Read the model definition and answer for the solid it produces. Units are mm, in the model's axes. A direction names the side the tool comes from. Coordinates: 2 decimals unless noted, no trailing zeros. Loops run counter-clockwise (first coordinate to the right, second up) from the corner with the lowest first, then second, coordinate; pieces in that order, holes last. Notation, with made-up numbers: (-33.5, 58.25) -> (-0.5, 58.25) arc R19 cw to (-0.5, 91.25) -> close; hole circle Ø3 at (71.25, -14). An arc over 180 degrees is marked (long way). Answer as a JSON object with one key per item and string values. Group by question number.
1) Section C-C, the plane z = -61 is taken. Give the vertices of the cut face in (x, y).
2) Section A-A, the plane y = 6 is taken. Give the vertices of the cut face in (x, z).
3) Which of the six approach directions +Z, -Z, +X, -X, +Y, -Y give full straight-line access (tool end or side, diameter ignored) to faces 1 (the face through (17.656, 4.824, -16.21)), 2 (the face through (20.344, 4.824, -17.79)), 3 (the face through (20.344, 4.824, -50.79))?
4) Determine the mould class of faces 4 (the face through (28, 0, -33)), 5 (the face through (17.644, 4.824, -17.768)), 6 (the face through (17.644, 4.824, -50.768)) for opening direction Z: released by +Z, released by -Z, zero draft, split by the parting line, or undercut.
5) Section B-B, the plane x = 19 is taken. Give the vertices of the cut face in (y, z), plus the area to 3 significant figures.
6) Flat-ended cylindrical pins translate along their axes: P1, Ø0.5, axis at x = 18.5, y = 5, coming from the -Z side; P2, Ø0.9, axis at x = 19, y = 4, coming from the +Z side. Find the tip coordinate at first contact, or state that the pin passes through.
7) Consider probe 1 along Y at (x, z) = (51, -59); probe 2 along X at (y, z) = (3.5, -18.5). Determine where each line is inside the solid, lowest interval first. Write a range as [from, to].
8) Section D-D, the plane x = 13.5 is taken. Give the vertices of the cut face in (y, z), plus the area to 3 significant figures.
Autodesk Inventor part; units mm, degrees
ref_plane "YZ Plane" through (0, 0, 0) normal (1, 0, 0) x (0, 1, 0)
ref_plane "XZ Plane" through (0, 0, 0) normal (0, 1, 0) x (-1, 0, 0)
ref_plane "XY Plane" through (0, 0, 0) normal (0, 0, 1) x (1, 0, 0)
sketch "Sketch1" plane through (0, 0, 0) normal (0, 1, 0) x (-1, 0, 0)
  line L0 (0, 0) -> (-55, 0)
  line L1 (-55, 0) -> (-55, -67)
  line L2 (-55, -67) -> (0, -67)
  line L3 (0, -67) -> (0, 0)
  dimension "d0" = 55
  dimension "d1" = 67
extrude "Extrusion1" add sketch "Sketch1" along normal blind 3
sketch "Sketch2" plane through (0, 3, 0) normal (0, 1, 0) x (1, 0, 0)
  line L0 (55, 0) -> (55, 67)
  line L1 (0, 0) -> (55, 0)
  line L2 (20.8, 17) -> (19.9, 15.4412)
  line L3 (19.9, 15.4412) -> (18.1, 15.4412)
  line L4 (18.1, 15.4412) -> (17.2, 17)
  line L5 (17.2, 17) -> (18.1, 18.5588)
  line L6 (18.1, 18.5588) -> (19.9, 18.5588)
  line L7 (19.9, 18.5588) -> (20.8, 17)
  line L8 (20.8, 50) -> (19.9, 48.4412)
  line L9 (19.9, 48.4412) -> (18.1, 48.4412)
  line L10 (18.1, 48.4412) -> (17.2, 50)
  line L11 (17.2, 50) -> (18.1, 51.5588)
  line L12 (18.1, 51.5588) -> (19.9, 51.5588)
  line L13 (19.9, 51.5588) -> (20.8, 50)
  point P0 (19, 17)
  point P1 (19, 50)
extrude "Extrusion2" add sketch "Sketch2" along normal blind 3.7
properties part number "Star_Wars_Base"
Determined:
{
 "1": {"outline": "(0, 0) -> (55, 0) -> (55, 3) -> (0, 3) -> close"},
 "2": {"outline": "(17.2, -50) -> (18.1, -51.56) -> (19.9, -51.56) -> (20.8, -50) -> (19.9, -48.44) -> (18.1, -48.44) -> close; (17.2, -17) -> (18.1, -18.56) -> (19.9, -18.56) -> (20.8, -17) -> (19.9, -15.44) -> (18.1, -15.44) -> close"},
 "3": {"face 1": "+Z, -X, +Y", "face 2": "+X, +Y", "face 3": "-Z, +X, +Y"},
 "4": {"face 4": "zero draft", "face 5": "undercut", "face 6": "released by -Z"},
 "5": {"outline": "(0, -67) -> (3, -67) -> (3, -51.56) -> (6.7, -51.56) -> (6.7, -48.44) -> (3, -48.44) -> (3, -18.56) -> (6.7, -18.56) -> (6.7, -15.44) -> (3, -15.44) -> (3, 0) -> (0, 0) -> close", "area": "224 mm²"},
 "6": {"P1": "z = -51.56", "P2": "z = -15.44"},
 "7": {"probe 1": "[0, 3]", "probe 2": "[18.07, 19.93]"},
 "8": {"outline": "(0, -67) -> (3, -67) -> (3, 0) -> (0, 0) -> close", "area": "201 mm²"}
}
